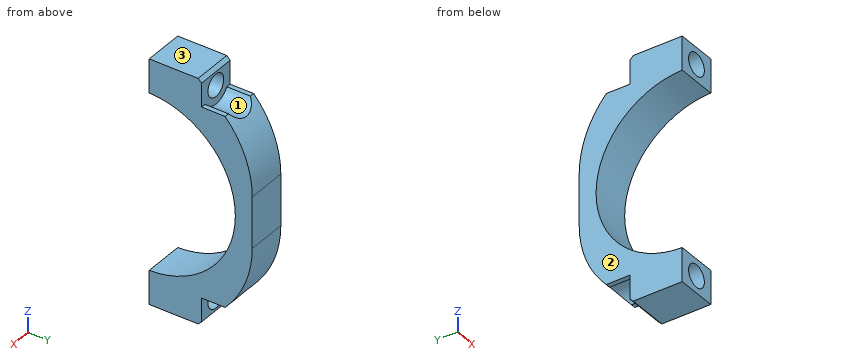
```python
from build123d import *

# Parameters (mm, degrees)
BOSS_EXTRUDE1_DEPTH  = 12
CHAMFER1_SIZE        = 16
FILLET1_R            = 30
M6_CLEARANCE_HOLE1_D = 6.6
SKETCH4_R            = 5.5
CUT_EXTRUDE1_DEPTH   = 15
SKETCH5_W            = 23.874068734
SKETCH5_H            = 12.946873537
CUT_EXTRUDE2_DEPTH   = 15


with BuildPart() as part:
    # Sketch1 → Boss-Extrude1 (new body)
    with BuildSketch(Plane(origin=(0, 0, 0), x_dir=(0, 0, -1), z_dir=(1, 0, 0))):
        with BuildLine():
            Line((-35.995191863, 0), (35.995191863, 0))
            Line((35.995191863, 0), (35.995191863, -30.5))
            Line((35.995191863, -30.5), (25.995191863, -30.5))
            ThreePointArc((25.995191863, -30.5), (0, -5), (-25.995191863, -30.5))
            Line((-25.995191863, -30.5), (-35.995191863, -30.5))
            Line((-35.995191863, -30.5), (-35.995191863, 0))
        make_face()
    extrude(amount=BOSS_EXTRUDE1_DEPTH)

    # Chamfer1
    chamfer1_edges = [part.edges().sort_by_distance(p)[0] for p in [
        (6, 0, 35.995191863),
        (6, 0, -35.995191863),
    ]]
    chamfer(chamfer1_edges, length=CHAMFER1_SIZE)

    # Fillet1
    fillet1_edges = [part.edges().sort_by_distance(p)[0] for p in [
        (6, 0, 19.995191863),
        (6, 0, -19.995191863),
    ]]
    fillet(fillet1_edges, radius=FILLET1_R)

    # M6 Clearance Hole1 (through all)
    with Locations(Plane(origin=(0, -30.5, 0), x_dir=(-1, 0, 0), z_dir=(0, -1, 0))):
        with Locations((-6, -30.995191863), (-6, 30.995191863)):
            Hole(M6_CLEARANCE_HOLE1_D / 2)

    # Sketch4 → Cut-Extrude1 (cut)
    with BuildSketch(Plane(origin=(0, 0, 0), x_dir=(1, 0, 0), z_dir=(0, 1, 0))):
        with Locations((6, -30.995191863)):
            Circle(SKETCH4_R)
        with Locations((6, 30.995191863)):
            Circle(SKETCH4_R)
    extrude(amount=-CUT_EXTRUDE1_DEPTH, mode=Mode.SUBTRACT)

    # Sketch5 → Cut-Extrude2 (cut)
    with BuildSketch(Plane(origin=(0, 0, 0), x_dir=(1, 0, 0), z_dir=(0, 1, 0))):
        with Locations((6, -34.473436769)):
            Rectangle(SKETCH5_W, SKETCH5_H)
        with Locations((6, 34.473436769)):
            Rectangle(SKETCH5_W, SKETCH5_H)
    extrude(amount=-CUT_EXTRUDE2_DEPTH, mode=Mode.SUBTRACT)


solid = part.part
```
Verification items for the finished model (mm, model axes). Face numbers are marked on the shaded views. Coordinates: 2 decimals unless noted, no trailing zeros. Loops run counter-clockwise (first coordinate to the right, second up) from the corner with the lowest first, then second, coordinate; pieces in that order, holes last. Notation, with made-up numbers: (78, 88.5) -> (102, 88.5) arc R33 cw to (102, 127.5) -> close; hole circle Ø10 at (-6.75, 55.5). An arc over 180 degrees is marked (long way). Put each result on its own line as item: value.
1. Section check B-B, the plane y = -21.5. Record the boundary of the cut face in (x, z), then the cut area to 3 significant figures.
Result set:
outline: (0, -36) -> (12, -36) -> (12, -24.2) -> (0, -24.2) -> close; (0, 24.2) -> (12, 24.2) -> (12, 36) -> (0, 36) -> close; hole circle Ø6.6 at (6, -31); hole circle Ø6.6 at (6, 31)
area: 215 mm^2
2. Gauge pin test, flat ends, axial feed: P1, Ø1.1, axis at x = 1, y = -13, coming from the +Z side; P2, Ø3, axis at x = 5.5, z = -10.5, coming from the -Y side; P3, Ø5, axis at x = 4.5, z = -28, coming from the +Y side; P4, Ø1, axis at y = -4, z = 4.5, coming from the -X side. Record the tip position at first contact, or that the pin passes through.
Result set:
P1: stops at z = 28
P2: stops at y = -7.93
P3: stops at y = -5.95
P4: stops at x = 0
3. Section check C-C, the plane z = -29. Record the boundary of the cut face in (x, y), then the cut area to 3 significant figures.
Result set:
outline: (0, -30.5) -> (3.37, -30.5) -> (3.37, -15) -> (0, -15) -> close; (8.63, -30.5) -> (12, -30.5) -> (12, -15) -> (8.63, -15) -> close
area: 105 mm^2
4. Mould release check, pull along X, two halves, no side actions. Record for the marked faces 1, 2 and 3: pulls with the +X half, pulls with the -X half, needs draft (parallel to the pull), parting line crosses it, or undercut.
Result set:
face 1: undercut
face 2: pulls with the -X half
face 3: needs draft
5. Thickness scan on line 1 (Z direction, x = 6, y = -20.75); line 2 (Z direction, x = 5, y = -27); line 3 (Z direction, x = 5.25, y = -10). Record the ranges inside material, lowest first.
Result set:
line 1: z = -36 to -34.3, -27.7 to -23.89, 23.89 to 27.7, 34.3 to 36
line 2: z = -36 to -34.14, -27.85 to -25.69, 25.69 to 27.85, 34.14 to 36
line 3: z = -25.55 to -15.33, 15.33 to 25.55
